Read the model definition and answer for the solid it produces. Units are mm, in the model's axes. Coordinates: 2 decimals unless noted, no trailing zeros. Loops run counter-clockwise (first coordinate to the right, second up) from the corner with the lowest first, then second, coordinate; pieces in that order, holes last. Notation, with made-up numbers: (-18.75, 6) - (11.25, 6) arc R12 cw to (11.25, 24) - close; hole circle Ø4 at (-6.75, 88). An arc over 180 degrees is marked (long way). Use one line per item in the form item = value. Start each with the question number.
1) A cutting plane is placed at A-A (y = 44.5). Give the vertices of the cut face in (x, z).
2) Each of these flat-tipped pins is pushed along its axis until it touches: P1, Ø1, axis at x = -44, z = 0.5, coming from the +Y side; P2, Ø0.6, axis at y = 80, z = 1.5, coming from the +X side. Where does it stop, or does it pass through?
3) Consider line 1 (X direction, y = 79, z = 1.6); line 2 (Y direction, x = 38, z = 0.7); line 3 (Y direction, x = 50.5, z = 0.85). Determine where each line is inside the solid, lowest interval first.
4) A cutting plane is placed at B-B (z = 1.6). State how many separate pieces and enclosed holes the cut face has, and give its area (3 significant figures).
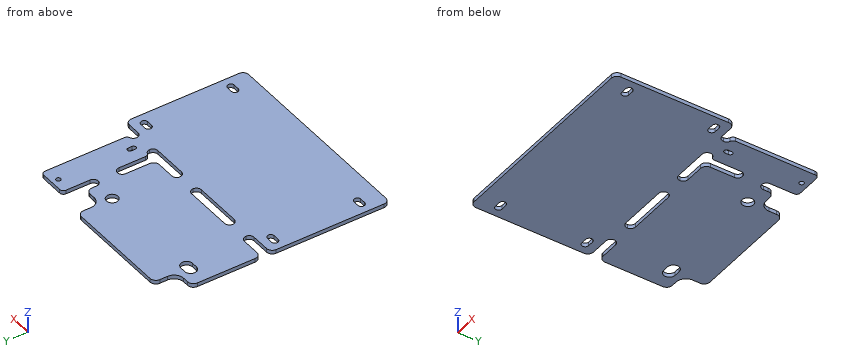
from build123d import *

# Parameters (mm, degrees)
SKETCH_1_W          = 110
SKETCH_1_H          = 65
EXTRUDE_1_DEPTH     = 2
FILLET_1_R          = 3
SKETCH_2_R          = 3
EXTRUDE_2_DEPTH     = 2
FILLET_5_R          = 3
FILLET_6_R          = 5
SKETCH_4_W          = 10
SKETCH_4_H          = 5
EXTRUDE_4_DEPTH     = 2
FILLET_7_R          = 2.5
SKETCH_5_W          = 16
SKETCH_5_H          = 45
SKETCH_5_R          = 1.2
EXTRUDE_5_DEPTH     = 2
SKETCH_6_W          = 10
SKETCH_6_H          = 5
SKETCH_6_W_2        = 5
SKETCH_6_H_2        = 10
EXTRUDE_6_DEPTH     = 2
FILLET_8_R          = 2.5
FILLET_9_R          = 2
SKETCH_7_W          = 110
SKETCH_7_H          = 3
CUT_EXTRUDE_1_DEPTH = 10
FILLET_10_R         = 3


with BuildPart() as part:
    # Sketch 1 → Extrude 1 (new body)
    with BuildSketch(Plane.XY):
        Rectangle(SKETCH_1_W, SKETCH_1_H)
        with BuildLine():
            Line((-49.5, 24.75), (-46.5, 24.75))
            ThreePointArc((-46.5, 24.75), (-44.75, 26.5), (-46.5, 28.25))
            Line((-46.5, 28.25), (-49.5, 28.25))
            ThreePointArc((-49.5, 28.25), (-51.25, 26.5), (-49.5, 24.75))
        make_face(mode=Mode.SUBTRACT)
        with BuildLine():
            Line((-46.5, -20.25), (-49.5, -20.25))
            ThreePointArc((-49.5, -20.25), (-51.25, -18.5), (-49.5, -16.75))
            Line((-49.5, -16.75), (-46.5, -16.75))
            ThreePointArc((-46.5, -16.75), (-44.75, -18.5), (-46.5, -20.25))
        make_face(mode=Mode.SUBTRACT)
        with BuildLine():
            Line((46.5, -20.25), (49.5, -20.25))
            ThreePointArc((49.5, -20.25), (51.25, -18.5), (49.5, -16.75))
            Line((49.5, -16.75), (46.5, -16.75))
            ThreePointArc((46.5, -16.75), (44.75, -18.5), (46.5, -20.25))
        make_face(mode=Mode.SUBTRACT)
        with BuildLine():
            Line((46.5, 28.25), (49.5, 28.25))
            ThreePointArc((49.5, 28.25), (51.25, 26.5), (49.5, 24.75))
            Line((49.5, 24.75), (46.5, 24.75))
            ThreePointArc((46.5, 24.75), (44.75, 26.5), (46.5, 28.25))
        make_face(mode=Mode.SUBTRACT)
    extrude(amount=EXTRUDE_1_DEPTH)

    # Fillet 1
    fillet_1_edges = [part.edges().sort_by_distance(p)[0] for p in [
        (-55, 32.5, 1),
        (55, 32.5, 1),
    ]]
    fillet(fillet_1_edges, radius=FILLET_1_R)



with BuildPart() as body_2:
    # Sketch 2 → Extrude 2 (new body)
    with BuildSketch(Plane.XY.offset(2)):
        Polygon((-55, 37.5), (25, 37.5), (25, 73.5), (14, 73.5), (14, 85.5), (-44, 85.5), (-44, 73.5), (-55, 73.5), align=None)
        with Locations((14, 67.5)):
            Circle(SKETCH_2_R, mode=Mode.SUBTRACT)
        with BuildLine():
            Line((-45.5, 64.5), (-42.5, 64.5))
            ThreePointArc((-42.5, 64.5), (-39.5, 67.5), (-42.5, 70.5))
            Line((-42.5, 70.5), (-45.5, 70.5))
            ThreePointArc((-45.5, 70.5), (-48.5, 67.5), (-45.5, 64.5))
        make_face(mode=Mode.SUBTRACT)
    extrude(amount=-EXTRUDE_2_DEPTH)

    # Fillet 5
    fillet_5_edges = [body_2.edges().sort_by_distance(p)[0] for p in [
        (25, 37.5, 1),
        (-55, 37.5, 1),
        (-55, 73.5, 1),
        (-44, 85.5, 1),
        (14, 85.5, 1),
        (25, 73.5, 1),
    ]]
    fillet(fillet_5_edges, radius=FILLET_5_R)

    # Fillet 6
    fillet_6_edges = [body_2.edges().sort_by_distance(p)[0] for p in [
        (-44, 73.5, 1),
        (14, 73.5, 1),
    ]]
    fillet(fillet_6_edges, radius=FILLET_6_R)


with BuildPart() as part_1:
    add(part.part)

    add(body_2.part)  # Extrude 4 merges body 2
    # Sketch 4 → Extrude 4 (add)
    with BuildSketch(Plane.XY.offset(2)):
        with Locations((-35, 35)):
            Rectangle(SKETCH_4_W, SKETCH_4_H)
        with Locations((5, 35)):
            Rectangle(SKETCH_4_W, SKETCH_4_H)
    extrude(amount=-EXTRUDE_4_DEPTH)

    # Fillet 7
    fillet_7_edges = [part_1.edges().sort_by_distance(p)[0] for p in [
        (10, 37.5, 1),
        (10, 32.5, 1),
        (0, 37.5, 1),
        (0, 32.5, 1),
        (-30, 37.5, 1),
        (-30, 32.5, 1),
        (-40, 37.5, 1),
        (-40, 32.5, 1),
    ]]
    fillet(fillet_7_edges, radius=FILLET_7_R - 0.0001)  # a hair under: the kernel refuses the full size



with BuildPart() as body_2_2:
    # Sketch 5 → Extrude 5 (new body)
    with BuildSketch(Plane.XY.offset(2)):
        with Locations((38, 60)):
            Rectangle(SKETCH_5_W, SKETCH_5_H)
        with Locations((38, 79)):
            Circle(SKETCH_5_R, mode=Mode.SUBTRACT)
        with BuildLine():
            Line((36.683223365, 42), (36.683223365, 40))
            ThreePointArc((36.683223365, 40), (37.883223365, 38.8), (39.083223365, 40))
            Line((39.083223365, 40), (39.083223365, 42))
            ThreePointArc((39.083223365, 42), (37.883223365, 43.2), (36.683223365, 42))
        make_face(mode=Mode.SUBTRACT)
    extrude(amount=-EXTRUDE_5_DEPTH)


with BuildPart() as part_2:
    add(part_1.part)

    add(body_2_2.part)  # Extrude 6 merges body 2 2
    # Sketch 6 → Extrude 6 (add)
    with BuildSketch(Plane.XY.offset(2)):
        with Locations((38, 35)):
            Rectangle(SKETCH_6_W, SKETCH_6_H)
        with Locations((27.5, 60.5)):
            Rectangle(SKETCH_6_W_2, SKETCH_6_H_2)
    extrude(amount=-EXTRUDE_6_DEPTH)

    # Fillet 8
    fillet_8_edges = [part_2.edges().sort_by_distance(p)[0] for p in [
        (43, 32.5, 1),
        (43, 37.5, 1),
        (33, 32.5, 1),
        (33, 37.5, 1),
        (30, 55.5, 1),
        (25, 55.5, 1),
        (25, 65.5, 1),
        (30, 65.5, 1),
    ]]
    fillet(fillet_8_edges, radius=FILLET_8_R - 0.0001)  # a hair under: the kernel refuses the full size

    # Fillet 9
    fillet_9_edges = [part_2.edges().sort_by_distance(p)[0] for p in [
        (46, 82.5, 1),
        (30, 82.5, 1),
        (46, 37.5, 1),
        (30, 37.5, 1),
    ]]
    fillet(fillet_9_edges, radius=FILLET_9_R)

    # Sketch 7 → Cut-Extrude 1 (cut)
    with BuildSketch(Plane.XY.offset(2)):
        with Locations((0, -31)):
            Rectangle(SKETCH_7_W, SKETCH_7_H)
    extrude(amount=-CUT_EXTRUDE_1_DEPTH, mode=Mode.SUBTRACT)

    # Fillet 10
    fillet_10_edges = [part_2.edges().sort_by_distance(p)[0] for p in [
        (55, -29.5, 1),
        (-55, -29.5, 1),
    ]]
    fillet(fillet_10_edges, radius=FILLET_10_R)


solid = part_2.part
Found:
q1.outline = (-55, 0) - (25, 0) - (25, 2) - (-55, 2) - close; (30, 0) - (46, 0) - (46, 2) - (30, 2) - close
q2.P1 = 84.16
q2.P2 = 46
q3.line_1 = -44 to 14, 30 to 36.8, 39.2 to 46
q3.line_2 = -29.5 to 38.81, 43.19 to 77.8, 80.2 to 82.5
q3.line_3 = -29.5 to -19.94, -17.06 to 25.06, 27.94 to 32.5
q4.separate_pieces = 1
q4.enclosed_holes = 10
q4.area = 11,200 mm^2
